Can you work these out from the model? Positions are in its coordinate system, mm. A direction names the side the tool comes from. Give positions to 0.01 mm unless a question says otherwise; leave off trailing zeros. Order: outer loops, then holes, each group sorted by start corner. A loop starts at its lowest first (then second) coordinate and runs counter-clockwise, first axis right, second up.
Item 1: Which directions (+Z, -Z, +X, -X, +Y, -Y) give clear straight access to the entire face, cutting with the end or side of a thin tool? Please do faces 4 (the cylindrical face through (-69.894, 5.183, 14.602)), 5 (the cylindrical face through (-27.95, 6.44, -0.11)), 6 (the cylindrical face through (69.894, 5.183, 14.602)).
Item 2: If we mould it in two halves opening along Y, with no side actions, what happens to faces 1 (the flat face through (-1, 0, -5)), 2 (the flat face through (-1, 6, 22.225)), 3 (the cylindrical face through (69.894, 5.183, -17.148))? For each: +Y half, -Y half, draft (parallel to the pull), parting line (faces both ways), or undercut.
Item 3: I'm going to push a flat-ended pin straight in: pin 1 Ø2 at (y, z) = (6.35, -15.875) entering from -X. Where does the tip first touch, or does it pass through?
Item 4: If I drill on line 1 along Z through (x, y) = (69.5, 6.35) (3 decimals); line 2 along Z through (x, y) = (-2, 8) (3 decimals); line 3 along X through (y, z) = (5.75, -16.5), over which ranges is the centre line in solid material (lowest first)?
Item 5: I want a section at B-B, the plane z = 0. Write out the boundary of the cut face in (x, y) (3 decimals), then the cut area to 3 significant figures.
Item 6: I want a section at A-A, the plane x = 25.4. Write out the boundary of the cut face in (y, z) (3 decimals).
```python
from build123d import *

# Parameters (mm, degrees)
SKETCH2_W                      = 146.05
SKETCH2_H                      = 44.45
BOSS_EXTRUDE1_DEPTH            = 12.7
F_1_4_20_TAPPED_HOLE1_D        = 5.1054
F_8_32_TAPPED_HOLE1_AT_2_COUNT = 2
F_8_32_TAPPED_HOLE1_AT_2_PITCH = 31.75


with BuildPart() as part:
    # Sketch2 → Boss-Extrude1 (new body)
    with BuildSketch(Plane(origin=(0, 0, 0), x_dir=(1, 0, 0), z_dir=(0, 1, 0))):
        Rectangle(SKETCH2_W, SKETCH2_H)
    extrude(amount=BOSS_EXTRUDE1_DEPTH)

    # 1/4-20 Tapped Hole1 (through all)
    with Locations(Plane(origin=(0, 0, 0), x_dir=(-1, 0, 0), z_dir=(0, -1, 0))):
        with Locations((0, 0), (-25.4, 0), (25.4, 0)):
            Hole(F_1_4_20_TAPPED_HOLE1_D / 2)

    # Sketch7 → #8-32 Tapped Hole1 (revolve, cut)
    with BuildSketch(Plane(origin=(-73.025, 6.35, -15.875), x_dir=(0, 0, 1), z_dir=(0, 1, 0))):
        Polygon((0, 0), (0, 7.387806461), (1.7272, 6.35), (1.7272, 0), align=None)
    f_8_32_tapped_hole1 = revolve(axis=Axis((-79.375, 6.35, -15.875), (1, 0, 0)), mode=Mode.SUBTRACT)

    # #8-32 Tapped Hole1 at 2: #8-32 Tapped Hole1 ×2
    with Locations(*[(0, 0, i * F_8_32_TAPPED_HOLE1_AT_2_PITCH) for i in range(1, F_8_32_TAPPED_HOLE1_AT_2_COUNT)]):
        add(f_8_32_tapped_hole1, mode=Mode.SUBTRACT)

    # Mirror1: #8-32 Tapped Hole1 across plane
    add(f_8_32_tapped_hole1.mirror(Plane(origin=(0, 0, 0), x_dir=(0, 0, 1), z_dir=(1, 0, 0))), mode=Mode.SUBTRACT)

    # Mirror1 copy 1 sketch → Mirror1 copy 1 (revolve, cut)
    with BuildSketch(Plane(origin=(73.025, 6.35, 15.875), x_dir=(0, 0, 1), z_dir=(0, 1, 0))):
        Polygon((0, 0), (0, -7.387806461), (1.7272, -6.35), (1.7272, 0), align=None)
    revolve(axis=Axis((79.375, 6.35, 15.875), (1, 0, 0)), mode=Mode.SUBTRACT)


solid = part.part
```
Results list:
1. face 4: -X
1. face 5: +Y, -Y
1. face 6: +X
2. face 1: -Y half
2. face 2: draft
2. face 3: undercut
3. pin 1: stops at x = -66.24
4. line 1: z = -22.225 to -17.602, -14.148 to 14.148, 17.602 to 22.225
4. line 2: z = -22.225 to -1.586, 1.586 to 22.225
4. line 3: x = -66.16 to 66.16
5. outline: (-73.025, 0) - (-27.953, 0) - (-27.953, 12.7) - (-73.025, 12.7) - close; (-22.847, 0) - (-2.553, 0) - (-2.553, 12.7) - (-22.847, 12.7) - close; (2.553, 0) - (22.847, 0) - (22.847, 12.7) - (2.553, 12.7) - close; (27.953, 0) - (73.025, 0) - (73.025, 12.7) - (27.953, 12.7) - close
5. area: 1,660 mm2
6. outline: (0, -22.225) - (12.7, -22.225) - (12.7, -2.553) - (0, -2.553) - close; (0, 2.553) - (12.7, 2.553) - (12.7, 22.225) - (0, 22.225) - close
